from build123d import *

# Parameters (mm, degrees)
SALIENTE_EXTRUIR1_DEPTH = 20
SALIENTE_EXTRUIR2_DEPTH = 20
CORTAR_EXTRUIR2_REACH   = 89.477
CROQUIS4_R              = 3
REDONDEO1_R             = 5
CORTAR_EXTRUIR3_REACH   = 86.815
CROQUIS5_R              = 3


with BuildPart() as part:
    # Croquis1 → Saliente-Extruir1 (new body)
    with BuildSketch(Plane.XY):
        with BuildLine():
            Line((0, -20.75), (25, -20.75))
            ThreePointArc((25, -20.75), (34.287921033, -18.054172905), (40, -10.25))
            Line((40, -10.25), (40, -6.25))
            Line((40, -6.25), (40, -2.25))
            ThreePointArc((40, -2.25), (34.287921033, 5.554172905), (25, 8.25))
            Line((25, 8.25), (0, 8.25))
            ThreePointArc((0, 8.25), (-9.287921033, 5.554172905), (-15, -2.25))
            Line((-15, -2.25), (-15, -6.25))
            Line((-15, -6.25), (-15, -10.25))
            ThreePointArc((-15, -10.25), (-9.287921033, -18.054172905), (0, -20.75))
        make_face()
        with BuildLine():
            Line((0, 3.25), (25, 3.25))
            ThreePointArc((25, 3.25), (31.967514421, 0.571067812), (35, -6.25))
            ThreePointArc((35, -6.25), (31.967514421, -13.071067812), (25, -15.75))
            Line((25, -15.75), (0, -15.75))
            ThreePointArc((0, -15.75), (-6.967514421, -13.071067812), (-10, -6.25))
            ThreePointArc((-10, -6.25), (-6.967514421, 0.571067812), (0, 3.25))
        make_face(mode=Mode.SUBTRACT)
    extrude(amount=SALIENTE_EXTRUIR1_DEPTH)

    # Croquis3 → Saliente-Extruir2 (add, through all)
    with BuildSketch(Plane.XY.offset(20)):
        with BuildLine():
            Line((40, -10.25), (40, -35.25))
            Line((40, -35.25), (70, -35.25))
            Line((70, -35.25), (70, -40.25))
            Line((70, -40.25), (40, -40.25))
            Line((40, -40.25), (-15, -40.25))
            Line((-15, -40.25), (-45, -40.25))
            Line((-45, -40.25), (-45, -35.25))
            Line((-45, -35.25), (-15, -35.25))
            Line((-15, -35.25), (-15, -10.25))
            ThreePointArc((-15, -10.25), (-13.047109047, -14.26290739), (-10, -17.523633574))
            Line((-10, -17.523633574), (-10, -35.25))
            Line((-10, -35.25), (35, -35.25))
            Line((35, -35.25), (35, -17.523633574))
            ThreePointArc((35, -17.523633574), (38.047109047, -14.26290739), (40, -10.25))
        make_face()
    extrude(amount=-SALIENTE_EXTRUIR2_DEPTH)

    # Cortar-Extruir2: up to this face of the body (flat: up to its plane)
    cortar_extruir2_end = Plane(part.part.faces().sort_by_distance((12.5, -20.75, 10))[0])
    # Croquis4 → Cortar-Extruir2 (cut, up to the picked face)
    with BuildSketch(Plane(origin=(0, 8.25, 0), x_dir=(1, 0, 0), z_dir=(0, 1, 0)), mode=Mode.PRIVATE) as cortar_extruir2_sk1:
        with Locations(Location((12.5, -15, 0), (0, 0, 270))):
            Circle(CROQUIS4_R)
    cortar_extruir2_tool1 = split(extrude(cortar_extruir2_sk1.sketch, amount=-CORTAR_EXTRUIR2_REACH, mode=Mode.PRIVATE), bisect_by=cortar_extruir2_end, keep=Keep.BOTH, mode=Mode.PRIVATE)
    add(cortar_extruir2_tool1.solids().sort_by(Axis((12.5, 8.25, 15), (0, -1, 0)))[0], mode=Mode.SUBTRACT)

    # Redondeo1
    redondeo1_edges = [part.edges().sort_by_distance(p)[0] for p in [
        (70, -37.75, 0),
        (-45, -37.75, 0),
        (-45, -37.75, 20),
        (70, -37.75, 20),
    ]]
    fillet(redondeo1_edges, radius=REDONDEO1_R)

    # Croquis5 → Cortar-Extruir3 (cut, up to next)
    with BuildSketch(Plane(origin=(0, -35.25, 0), x_dir=(1, 0, 0), z_dir=(0, 1, 0)), mode=Mode.PRIVATE) as cortar_extruir3_sk1:
        with Locations(Location((-30, -10, 0), (0, 0, 180))):
            Circle(CROQUIS5_R)
    cortar_extruir3_tool1 = extrude(cortar_extruir3_sk1.sketch, amount=-CORTAR_EXTRUIR3_REACH, mode=Mode.PRIVATE) & part.part
    # Croquis5 → Cortar-Extruir3 (cut, up to next)
    with BuildSketch(Plane(origin=(0, -35.25, 0), x_dir=(1, 0, 0), z_dir=(0, 1, 0)), mode=Mode.PRIVATE) as cortar_extruir3_sk2:
        with Locations(Location((55, -10, 0), (0, 0, 90))):
            Circle(CROQUIS5_R)
    cortar_extruir3_tool2 = extrude(cortar_extruir3_sk2.sketch, amount=-CORTAR_EXTRUIR3_REACH, mode=Mode.PRIVATE) & part.part
    add(cortar_extruir3_tool1.solids().sort_by_distance((-30, -35.25, 10))[0], mode=Mode.SUBTRACT)
    add(cortar_extruir3_tool2.solids().sort_by_distance((55, -35.25, 10))[0], mode=Mode.SUBTRACT)


solid = part.part
Here's how the part is built. I have some questions about the finished solid (model axes, mm). A direction names the side the tool comes from. Give positions to 0.01 mm unless a question says otherwise; leave off trailing zeros. Loops run counter-clockwise (first coordinate to the right, second up) from the corner with the lowest first, then second, coordinate; pieces in that order, holes last. Notation, with made-up numbers: (33.25, 23.25) -> (41.25, 23.25) arc R18 ccw to (41.25, 57.25) -> close; hole circle Ø11 at (63.5, -35.5). An arc over 180 degrees is marked (long way). One line per item, written item: value.
Q1. Suppose I cut it at A-A on x = 55. Please give me the cut outline in (y, z).
Answers follow:
outline: (-40.25, 0) -> (-35.25, 0) -> (-35.25, 7) -> (-40.25, 7) -> close; (-40.25, 13) -> (-35.25, 13) -> (-35.25, 20) -> (-40.25, 20) -> close
Q2. On a 3-axis mill with a long thin cutter (end or side, diameter ignored), from which of +Z, -Z, +X, -X, +Y, -Y can I reach the whole of each face in a straight line? I mean faces 1 (the face through (31.889, 0.645, 9.86)), 2 (the face through (-34, -35.25, 10)), 3 (the face through (51, -35.25, 10)). Say none if no direction works.
Answers follow:
face 1: +Z, -Z
face 2: +Z, -Z, -X, +Y
face 3: +Z, -Z, +X, +Y
Q3. I'm going to push flat-ended pins straight in: pin 1 Ø4 at (y, z) = (-19, 12.5) entering from -X; pin 2 Ø9.5 at (x, z) = (-30, 10) entering from -Y; pin 3 Ø5.5 at (y, z) = (-29, 10) entering from +X; pin 4 Ø6 at (x, z) = (52.5, 10) entering from +Y. Where does each tip first touch, or does it pass through?
Answers follow:
pin 1: x = -15
pin 2: y = -40.25
pin 3: x = 40
pin 4: y = -35.25
Q4. Suppose I cut it at D-D on z = 2.5. Please give me the cut outline in (x, y), then the cut area to 3 significant figures.
Answers follow:
outline: (-44.33, -40.25) -> (69.33, -40.25) -> (69.33, -35.25) -> (40, -35.25) -> (40, -2.25) arc R15 ccw to (25, 8.25) -> (0, 8.25) arc R15 ccw to (-15, -2.25) -> (-15, -35.25) -> (-44.33, -35.25) -> close; hole (-10, -35.25) -> (35, -35.25) -> (35, -17.52) arc R15 cw to (25, -20.75) -> (0, -20.75) arc R15 cw to (-10, -17.52) -> close; hole (-10, -6.25) arc R9.75 ccw to (0, -15.75) -> (25, -15.75) arc R9.75 ccw to (35, -6.25) arc R9.75 ccw to (25, 3.25) -> (0, 3.25) arc R9.75 ccw to start
area: 1,440 mm^2
Q5. Suppose I cut it at C-C on y = -33. Please give me the cut outline in (x, z), then the cut area to 3 significant figures.
Answers follow:
outline: (-15, 0) -> (-10, 0) -> (-10, 20) -> (-15, 20) -> close; (35, 0) -> (40, 0) -> (40, 20) -> (35, 20) -> close
area: 200 mm^2
Q6. We'd pull the mould along Y, two halves only. Please class faces 4 (the face through (34.4, 5.475, 9.86)), 5 (the face through (30.22, -20.064, 9.86)), 6 (the face through (-6.889, -13.145, 9.86)), 7 (the face through (68, -38, 1)): pulls with the +Y half, pulls with the -Y half, needs draft (parallel to the pull), parting line crosses it, or undercut.
Answers follow:
face 4: pulls with the +Y half
face 5: undercut
face 6: undercut
face 7: needs draft
Q7. Suppose I cut it at B-B on z = 10. State how many separate pieces and enclosed holes the cut face has, then the cut area to 3 significant figures.
Answers follow:
separate pieces: 3
enclosed holes: 2
area: 1,380 mm^2
Q8. If I drill on line 1 along Y through (x, z) = (10, 4.5); line 2 along Y through (x, z) = (-5.5, 6.25); line 3 along X through (y, z) = (-19.6, 15), over which ranges is the centre line in solid material (lowest first)?
Answers follow:
line 1: -40.25 to -35.25, -20.75 to -15.75, 3.25 to 8.25
line 2: -40.25 to -35.25, -19.97 to -14.22, 1.72 to 7.47
line 3: -15 to -10, -6.48 to 9.5, 15.5 to 31.48, 35 to 40
